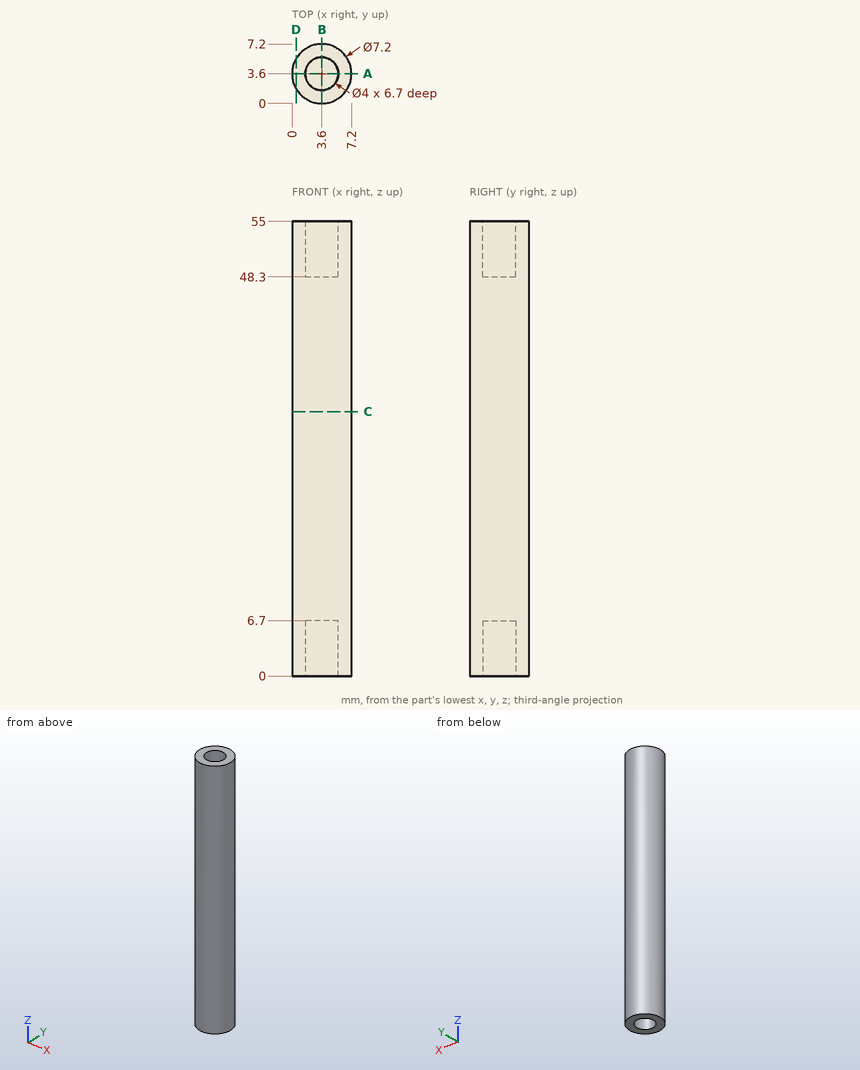
Drawing for the job (mm, zero at the part's lowest x, y, z). Give positions to 0.01 mm unless a question says otherwise; leave off trailing zeros. Order: outer loops, then holes, each group sorted by start corner. A loop starts at its lowest first (then second) coordinate and runs counter-clockwise, first axis right, second up. Notation, with made-up numbers: (83.5, 54) - (139.5, 54) arc R13 cw to (139.5, 73) - close; hole circle Ø7 at (14.5, 31.5). An arc over 180 degrees is marked (long way). Use one line per item in the form item = value.
Item 1: Pin check, flat tips, straight feed: pin 1 Ø3 at (x, y) = (3.6, 3.6) entering from -Z; pin 2 Ø2 at (x, z) = (5.5, 48) entering from -Y; pin 3 Ø1.2 at (x, y) = (4, 3.5) entering from +Z; pin 4 Ø3 at (x, y) = (4, 4) entering from -Z. Stop position of each tip, or through.
Solution:
pin_1 = 6.7
pin_2 = 0.11
pin_3 = 48.3
pin_4 = 0
Item 2: Slice it at C-C on z = 32. Give the cut face in (x, y), and give its area (3 significant figures).
Solution:
outline = circle Ø7.2 at (3.6, 3.6)
area = 40.7 mm2
Item 3: Probe probe 1 along Y at (x, z) = (3.6, 3); probe 2 along Z at (x, y) = (3.5, 3.5); probe 3 along Y at (x, z) = (5, 21.5). List the from-to ranges inside material, lowest first. Write a range as from..to.
Solution:
probe_1 = 0..1.6, 5.6..7.2
probe_2 = 6.7..48.3
probe_3 = 0.28..6.92
Item 4: Slice it at D-D on x = 0.5. Give the cut face in (y, z), and give its area (3 significant figures).
Solution:
outline = (1.77, 0) - (5.43, 0) - (5.43, 55) - (1.77, 55) - close
area = 201 mm2
Item 5: Slice it at A-A on y = 3.6. Give the cut face in (x, z), and give its area (3 significant figures).
Solution:
outline = (0, 0) - (1.6, 0) - (1.6, 6.7) - (5.6, 6.7) - (5.6, 0) - (7.2, 0) - (7.2, 55) - (5.6, 55) - (5.6, 48.3) - (1.6, 48.3) - (1.6, 55) - (0, 55) - close
area = 342 mm2
